The listing builds one solid part. Answer for the finished solid, in the listing's coordinates (mm). A direction names the side the tool comes from. Coordinates: 2 decimals unless noted, no trailing zeros. Order: outer loops, then holes, each group sorted by start corner. A loop starts at its lowest first (then second) coordinate and runs counter-clockwise, first axis right, second up. Notation, with made-up numbers: (-17, 51.5) - (41, 51.5) arc R14 ccw to (41, 77.5) - close; hole circle Ø3 at (80, 45). An arc over 180 degrees is marked (long way). Use one line per item in the form item = value. Start each with the question number.
Item 1: Section A-A, the plane x = 0 is taken. Write down the section's boundary in (y, z), and give its area (3 significant figures).
Item 2: A tool of negligible diameter and unlimited length cuts with its end or side. For faces 5 (the cylindrical face through (6.7, 4.44, -0.81)), 6 (the cylindrical face through (5.56, 4.44, -3.83)), 7 (the cylindrical face through (-2.04, 4.44, -8.25)), 8 (the cylindrical face through (-3.945, 4.437, 7.529)), from which of +Z, -Z, +X, -X, +Y, -Y can it reach the whole face along a straight path? Write none if from no direction.
Item 3: Each of these flat-tipped pins is pushed along its axis until it touches: pin 1 Ø5 at (y, z) = (3, 6.5) entering from +X; pin 2 Ø5 at (x, y) = (-6, 0.5) entering from -Z; pin 3 Ø4 at (x, y) = (2, 3) entering from +Z. Where does it stop, or does it pass through?
Item 4: Section B-B, the plane y = -1.5 is taken. Write down the section's boundary in (x, z), and give its area (3 significant figures).
Item 5: Consider line 1 along X through (y, z) = (-2.5, 0); line 2 along Y through (x, z) = (5, 6.5); line 3 along Y through (x, z) = (1.5, 0.5). Determine where each line is inside the solid, lowest interval first. Write a range as [from, to].
Item 6: The mould has two halves that part along Z. Classify faces 1 (the cylindrical face through (0.691, -2.014, -2.194)), 2 (the cylindrical face through (6.31, 4.44, 2.4)), 3 (the cylindrical face through (-3.543, -1.479, -8.545)), 4 (the cylindrical face through (8.44, 4.44, 1.02)): released by +Z, released by -Z, zero draft, split by the parting line, or undercut.
from build123d import *

# Parameters (mm, degrees)
SKETCH1_R             = 0.4
BOSS_EXTRUDE1_DEPTH   = 9
SKETCH2_R             = 9.25
BOSS_EXTRUDE2_DEPTH   = 3
CROQUIS1_R            = 2.3
CORTAR_EXTRUIR1_DEPTH = 2


with BuildPart() as part:
    # Sketch1 → Boss-Extrude1 (new body)
    with BuildSketch(Plane(origin=(0, 0, 0), x_dir=(1, 0, 0), z_dir=(0, 1, 0))):
        with BuildLine():
            add(Edge.make_bspline(
                [(-5.065227978, 4.461610195), (-5.526615005, 4.86619147), (-5.830003112, 5.39406146), (-5.975392301, 6.045220165)],
                knots=[0, 0, 0, 0, 0.872429449, 0.872429449, 0.872429449, 0.872429449], degree=3))
            ThreePointArc((-5.065227978, 4.461610195), (-5.560258819, 3.827012132), (-5.976238464, 3.138004752))
            add(Edge.make_bspline(
                [(-7.780961116, 3.42149735), (-7.125870497, 3.507536778), (-6.52429628, 3.413039245), (-5.976238464, 3.138004752)],
                knots=[0.127683247, 0.127683247, 0.127683247, 0.127683247, 1, 1, 1, 1], degree=3))
            ThreePointArc((-7.780961116, 3.42149735), (-7.951879756, 3.00293329), (-8.10030101, 2.575873357))
            add(Edge.make_bspline(
                [(-6.558450277, 1.596630818), (-7.155006493, 1.740452504), (-7.668956737, 2.066866683), (-8.10030101, 2.575873357)],
                knots=[0, 0, 0, 0, 0.872429449, 0.872429449, 0.872429449, 0.872429449], degree=3))
            ThreePointArc((-6.558450277, 1.596630818), (-6.701865893, 0.804669837), (-6.749999881, 0.00126872))
            add(Edge.make_bspline(
                [(-8.479748007, -0.586407486), (-7.939678588, -0.205787566), (-7.363095879, -0.009895497), (-6.749999881, 0.00126872)],
                knots=[0.127683247, 0.127683247, 0.127683247, 0.127683247, 1, 1, 1, 1], degree=3))
            ThreePointArc((-8.479748007, -0.586407486), (-8.436572529, -1.036457408), (-8.369528376, -1.483574994))
            add(Edge.make_bspline(
                [(-6.549210655, -1.634117437), (-7.144272221, -1.784003157), (-7.751044795, -1.733822342), (-8.369528376, -1.483574994)],
                knots=[0, 0, 0, 0, 0.872429449, 0.872429449, 0.872429449, 0.872429449], degree=3))
            ThreePointArc((-6.549210655, -1.634117437), (-6.308156258, -2.402012621), (-5.977417671, -3.13575796))
            add(Edge.make_bspline(
                [(-7.235926822, -4.459973434), (-6.934601997, -3.871968458), (-6.515098947, -3.4305633), (-5.977417671, -3.13575796)],
                knots=[0.127683247, 0.127683247, 0.127683247, 0.127683247, 1, 1, 1, 1], degree=3))
            ThreePointArc((-7.235926822, -4.459973434), (-6.988548208, -4.838408204), (-6.721397655, -5.203154193))
            add(Edge.make_bspline(
                [(-5.039625799, -4.490509081), (-5.496871281, -4.899765193), (-6.0574619, -5.137313564), (-6.721397655, -5.203154193)],
                knots=[0, 0, 0, 0, 0.872429449, 0.872429449, 0.872429449, 0.872429449], degree=3))
            ThreePointArc((-5.039625799, -4.490509081), (-4.469324045, -5.058422935), (-3.835481109, -5.554420281))
            add(Edge.make_bspline(
                [(-4.334442004, -7.311813216), (-4.34089166, -6.651128039), (-4.174571361, -6.065330394), (-3.835481109, -5.554420281)],
                knots=[0.127683247, 0.127683247, 0.127683247, 0.127683247, 1, 1, 1, 1], degree=3))
            ThreePointArc((-4.334442004, -7.311813216), (-3.939531713, -7.53193799), (-3.533475733, -7.730753472))
            add(Edge.make_bspline(
                [(-2.375523406, -6.318179211), (-2.590203375, -6.893050073), (-2.976187484, -7.36390816), (-3.533475733, -7.730753472)],
                knots=[0, 0, 0, 0, 0.872429449, 0.872429449, 0.872429449, 0.872429449], degree=3))
            ThreePointArc((-2.375523406, -6.318179211), (-1.606623554, -6.556009515), (-0.814882047, -6.700631854))
            add(Edge.make_bspline(
                [(-0.439988759, -8.488604708), (-0.752735357, -7.906594341), (-0.877699786, -7.31060339), (-0.814882047, -6.700631854)],
                knots=[0.127683247, 0.127683247, 0.127683247, 0.127683247, 1, 1, 1, 1], degree=3))
            ThreePointArc((-0.439988759, -8.488604708), (0.011984021, -8.499991552), (0.463922896, -8.487330296))
            add(Edge.make_bspline(
                [(0.832782771, -6.698430626), (0.909848909, -7.307220251), (0.786895617, -7.903520141), (0.463922896, -8.487330296)],
                knots=[0, 0, 0, 0, 0.872429449, 0.872429449, 0.872429449, 0.872429449], degree=3))
            ThreePointArc((0.832782771, -6.698430626), (1.624135031, -6.551693323), (2.392396671, -6.311809421))
            add(Edge.make_bspline(
                [(3.555260608, -7.72075916), (3.007863545, -7.350755165), (2.620242233, -6.881105252), (2.392396671, -6.311809421)],
                knots=[0.127683247, 0.127683247, 0.127683247, 0.127683247, 1, 1, 1, 1], degree=3))
            ThreePointArc((3.555260608, -7.72075916), (3.96075436, -7.520799485), (4.355042381, -7.299562032))
            add(Edge.make_bspline(
                [(3.850308451, -5.54415231), (4.201465773, -6.047394331), (4.369710416, -6.632530905), (4.355042381, -7.299562032)],
                knots=[0, 0, 0, 0, 0.872429449, 0.872429449, 0.872429449, 0.872429449], degree=3))
            ThreePointArc((3.850308451, -5.54415231), (4.482823853, -5.046463148), (5.051606144, -4.477027515))
            add(Edge.make_bspline(
                [(6.736042616, -5.184180734), (6.079397157, -5.110946566), (5.517918333, -4.875228826), (5.051606144, -4.477027515)],
                knots=[0.127683247, 0.127683247, 0.127683247, 0.127683247, 1, 1, 1, 1], degree=3))
            ThreePointArc((6.736042616, -5.184180734), (7.002163607, -4.818682892), (7.24847414, -4.439552076))
            add(Edge.make_bspline(
                [(5.985774866, -3.119775513), (6.530577461, -3.402183249), (6.951477219, -3.84210877), (7.24847414, -4.439552076)],
                knots=[0, 0, 0, 0, 0.872429449, 0.872429449, 0.872429449, 0.872429449], degree=3))
            ThreePointArc((5.985774866, -3.119775513), (6.314551754, -2.385149082), (6.553553527, -1.616612559))
            add(Edge.make_bspline(
                [(8.373678438, -1.459968977), (7.758214146, -1.700281702), (7.151505842, -1.75249623), (6.553553527, -1.616612559)],
                knots=[0.127683247, 0.127683247, 0.127683247, 0.127683247, 1, 1, 1, 1], degree=3))
            ThreePointArc((8.373678438, -1.459968977), (8.439461558, -1.01266412), (8.481367828, -0.562494242))
            add(Edge.make_bspline(
                [(6.749972396, 0.019304256), (7.363612555, 0.022427015), (7.940744366, -0.171505818), (8.481367828, -0.562494242)],
                knots=[0, 0, 0, 0, 0.872429449, 0.872429449, 0.872429449, 0.872429449], degree=3))
            ThreePointArc((6.749972396, 0.019304256), (6.699691947, 0.822573894), (6.554160776, 1.614148852))
            add(Edge.make_bspline(
                [(8.093005444, 2.598704077), (7.65971777, 2.099897208), (7.146769547, 1.771712133), (6.554160776, 1.614148852)],
                knots=[0.127683247, 0.127683247, 0.127683247, 0.127683247, 1, 1, 1, 1], degree=3))
            ThreePointArc((8.093005444, 2.598704077), (7.943380571, 3.025343799), (7.771282357, 3.443424244))
            add(Edge.make_bspline(
                [(5.967832596, 3.153961653), (6.509732754, 3.44189952), (7.110882674, 3.53838705), (7.771282357, 3.443424244)],
                knots=[0, 0, 0, 0, 0.872429449, 0.872429449, 0.872429449, 0.872429449], degree=3))
            ThreePointArc((5.967832596, 3.153961653), (5.550013455, 3.841855105), (5.053288778, 4.475128213))
            add(Edge.make_bspline(
                [(5.958322434, 6.062045345), (5.806472362, 5.419014975), (5.504794477, 4.890042598), (5.053288778, 4.475128213)],
                knots=[0.127683247, 0.127683247, 0.127683247, 0.127683247, 1, 1, 1, 1], degree=3))
            ThreePointArc((5.958322434, 6.062045345), (5.627566824, 6.370281912), (5.280889753, 6.660495734))
            add(Edge.make_bspline(
                [(3.818534268, 5.566084444), (4.16455163, 6.072874324), (4.652003458, 6.437678087), (5.280889753, 6.660495734)],
                knots=[0, 0, 0, 0, 0.872429449, 0.872429449, 0.872429449, 0.872429449], degree=3))
            ThreePointArc((3.818534268, 5.566084444), (3.128893766, 5.98101361), (2.394769219, 6.310909632))
            add(Edge.make_bspline(
                [(2.45865956, 8.136645081), (2.623034112, 7.496701718), (2.601737332, 6.888123235), (2.394769219, 6.310909632)],
                knots=[0.127683247, 0.127683247, 0.127683247, 0.127683247, 1, 1, 1, 1], degree=3))
            ThreePointArc((2.45865956, 8.136645081), (2.022545337, 8.25586521), (1.580708948, 8.351727918))
            add(Edge.make_bspline(
                [(0.794455758, 6.703084368), (0.865321915, 7.312626807), (1.127406312, 7.862174657), (1.580708948, 8.351727918)],
                knots=[0, 0, 0, 0, 0.872429449, 0.872429449, 0.872429449, 0.872429449], degree=3))
            ThreePointArc((0.794455758, 6.703084368), (-0.009017778, 6.749993976), (-0.812363108, 6.700937709))
            add(Edge.make_bspline(
                [(-1.604252589, 8.347237485), (-1.161309642, 7.856984441), (-0.897346481, 7.308217849), (-0.812363108, 6.700937709)],
                knots=[0.127683247, 0.127683247, 0.127683247, 0.127683247, 1, 1, 1, 1], degree=3))
            ThreePointArc((-1.604252589, 8.347237485), (-2.045816912, 8.250129282), (-2.481593228, 8.129679886))
            add(Edge.make_bspline(
                [(-2.411622992, 6.304488444), (-2.632142622, 6.877144615), (-2.655466033, 7.485541762), (-2.481593228, 8.129679886)],
                knots=[0, 0, 0, 0, 0.872429449, 0.872429449, 0.872429449, 0.872429449], degree=3))
            ThreePointArc((-2.411622992, 6.304488444), (-3.144863458, 5.972632069), (-3.833392837, 5.555861712))
            add(Edge.make_bspline(
                [(-5.299649804, 6.645578377), (-4.679611352, 6.417326717), (-4.19085903, 6.054087828), (-3.833392837, 5.555861712)],
                knots=[0.127683247, 0.127683247, 0.127683247, 0.127683247, 1, 1, 1, 1], degree=3))
            ThreePointArc((-5.299649804, 6.645578377), (-5.645507162, 6.35438816), (-5.975392301, 6.045220165))
        make_face()
        with Locations(Location((0, 0, 0), (0, 0, 270))):
            Circle(SKETCH1_R, mode=Mode.SUBTRACT)
    extrude(amount=BOSS_EXTRUDE1_DEPTH)

    # Sketch2 → Boss-Extrude2 (add)
    with BuildSketch(Plane.XZ):
        with Locations(Location((0, 0, 0), (0, 0, 270))):
            Circle(SKETCH2_R)
    extrude(amount=BOSS_EXTRUDE2_DEPTH)

    # Croquis1 → Cortar-Extruir1 (cut)
    with BuildSketch(Plane.XZ.offset(3)):
        with Locations(Location((0, 0, 0), (0, 0, 270))):
            Circle(CROQUIS1_R)
    extrude(amount=-CORTAR_EXTRUIR1_DEPTH, mode=Mode.SUBTRACT)


solid = part.part
Response:
q1.outline = (-3, -9.25) - (0, -9.25) - (0, -6.75) - (9, -6.75) - (9, -0.4) - (0, -0.4) - (0, 0.4) - (9, 0.4) - (9, 8.5) - (0, 8.5) - (0, 9.25) - (-3, 9.25) - (-3, 2.3) - (-1, 2.3) - (-1, -2.3) - (-3, -2.3) - close
q1.area = 176 mm2
q2.face_5 = +X, +Y
q2.face_6 = +Y
q2.face_7 = -Z, -X, +Y
q2.face_8 = +Z, -X, +Y
q3.pin_1 = 7.25
q3.pin_2 = -8.54
q3.pin_3 = 8.5
q4.outline = circle Ø18.5 at (0, 0); hole circle Ø4.6 at (0, 0)
q4.area = 252 mm2
q5.line_1 = [-9.25, -2.3], [2.3, 9.25]
q5.line_2 = [-3, 0]
q5.line_3 = [-1, 9]
q6.face_1 = undercut
q6.face_2 = undercut
q6.face_3 = split by the parting line
q6.face_4 = released by +Z
